For this review, use the dimensioned drawing (mm, ordinates from the lowest corner) and the shaded views. Coordinates: 2 decimals unless noted, no trailing zeros. Write each loop counter-clockwise with the first axis right and the second up, starting at its lowest first coordinate (ties: lowest second). Pieces come first, ordered by that corner, then holes. Notation, with made-up numbers: (-28, 38.5) - (4, 38.5) arc R29 ccw to (4, 59.5) - close; hole circle Ø7 at (32, -36.75). An arc over 180 degrees is marked (long way). Answer as a JSON object with one key per item and string values.
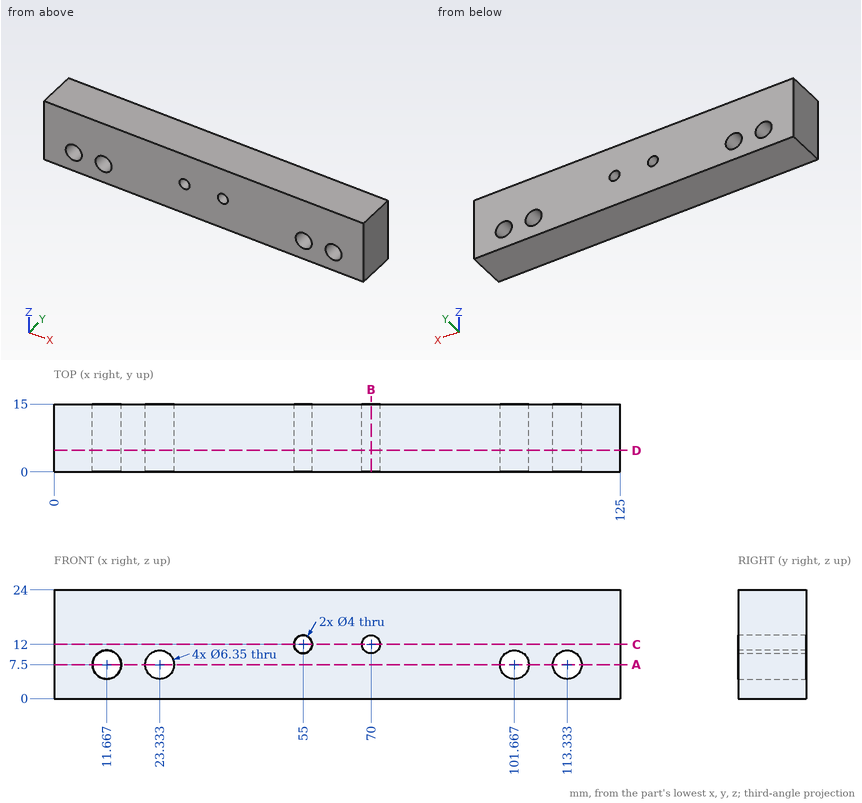
(1) Take a section at C-C, the plane z = 12. Write out the cut boundary in (x, y), and give its area (4 significant figures).
Solved:
{"outline": "(0, 0) - (53, 0) - (53, 15) - (0, 15) - close; (57, 0) - (68, 0) - (68, 15) - (57, 15) - close; (72, 0) - (125, 0) - (125, 15) - (72, 15) - close", "area": "1,755 mm^2"}
(2) Take a section at B-B, the plane x = 70. Write out the cut boundary in (y, z).
Solved:
{"outline": "(0, 0) - (15, 0) - (15, 10) - (0, 10) - close; (0, 14) - (15, 14) - (15, 24) - (0, 24) - close"}
(3) To check wall thickness, follow line 1 (X direction, y = 6, z = 7.5); line 2 (Z direction, x = 70, y = 6); line 3 (X direction, y = 10.5, z = 12). State the ranges of each line that lie inside material, in increasing order. Write a range as from..to.
Solved:
{"line 1": "x = 0..8.49, 14.84..20.16, 26.51..98.49, 104.84..110.16, 116.51..125", "line 2": "z = 0..10, 14..24", "line 3": "x = 0..53, 57..68, 72..125"}
(4) Take a section at D-D, the plane y = 4.75. Give the number of separate pieces and of enclosed holes in the cut face, and give its area (3 significant figures).
Solved:
{"separate pieces": "1", "enclosed holes": "6", "area": "2,850 mm^2"}
(5) Take a section at A-A, the plane z = 7.5. Write out the cut boundary in (x, y), and give its area (3 significant figures).
Solved:
{"outline": "(0, 0) - (8.49, 0) - (8.49, 15) - (0, 15) - close; (14.84, 0) - (20.16, 0) - (20.16, 15) - (14.84, 15) - close; (26.51, 0) - (98.49, 0) - (98.49, 15) - (26.51, 15) - close; (104.84, 0) - (110.16, 0) - (110.16, 15) - (104.84, 15) - close; (116.51, 0) - (125, 0) - (125, 15) - (116.51, 15) - close", "area": "1,490 mm^2"}
